```python
from build123d import *

# Parameters (mm, degrees)
SM_BASE_FLANGE_1_DEPTH = 113
EXTRUDE_1_DEPTH        = 4
HOLE_WIZARD_M3_1_D     = 2.5
SKETCH_10_R            = 11
CUT_EXTRUDE_1_DEPTH    = 2
HOLE_WIZARD_M3_2_D     = 2.5


# Sheet-metal steps are written as plain solids
with BuildPart() as part:
    # Sketch 1 → 基体-法兰1 (new body)
    with BuildSketch(Plane.XY):
        with BuildLine():
            Line((104, 47.58), (3.5, 47.58))
            ThreePointArc((3.5, 47.58), (1.025126266, 46.554873734), (0, 44.08))
            Line((0, 44.08), (0, -44.08))
            ThreePointArc((0, -44.08), (1.025126266, -46.554873734), (3.5, -47.58))
            Line((3.5, -47.58), (104, -47.58))
            Line((104, -47.58), (104, -45.58))
            Line((104, -45.58), (3.5, -45.58))
            ThreePointArc((3.5, -45.58), (2.439339828, -45.140660172), (2, -44.08))
            Line((2, -44.08), (2, 44.08))
            ThreePointArc((2, 44.08), (2.439339828, 45.140660172), (3.5, 45.58))
            Line((3.5, 45.58), (104, 45.58))
            Line((104, 45.58), (104, 47.58))
        make_face()
    extrude(amount=SM_BASE_FLANGE_1_DEPTH)

    # 草图6 → 凸台-拉伸1 (add)
    with BuildSketch(Plane.XY):
        with BuildLine():
            Line((104, 45.58), (3.5, 45.58))
            ThreePointArc((3.5, 45.58), (2.439339828, 45.140660172), (2, 44.08))
            Line((2, 44.08), (2, -44.08))
            ThreePointArc((2, -44.08), (2.439339828, -45.140660172), (3.5, -45.58))
            Line((3.5, -45.58), (104, -45.58))
            Line((104, -45.58), (104, 45.58))
        make_face()
    extrude(amount=EXTRUDE_1_DEPTH)

    # M3 螺纹孔1 (through all)
    with Locations(Plane(origin=(0, -47.58, 0), x_dir=(-1, 0, 0), z_dir=(0, -1, 0))):
        with Locations((-83.7, -100.6), (-96.2, -100.6)):
            Hole(HOLE_WIZARD_M3_1_D / 2)

    # 草图10 → 切除-拉伸1 (cut)
    with BuildSketch(Plane.ZY):
        with Locations(Location((47.4, -14.64, 0), (0, 0, 270))):
            Circle(SKETCH_10_R)
    extrude(amount=-CUT_EXTRUDE_1_DEPTH, mode=Mode.SUBTRACT)

    # M3 螺纹孔2 (through all)
    with Locations(Plane.XY.offset(4)):
        with Locations((41.5, 12.5), (66.5, 12.5), (66.5, -12.5), (41.5, -12.5)):
            Hole(HOLE_WIZARD_M3_2_D / 2)


solid = part.part
```
Geometry check sheet. Reference: the model listing, model coordinates, mm. A direction names the side the tool comes from. Give positions to 0.01 mm unless a question says otherwise; leave off trailing zeros. Order: outer loops, then holes, each group sorted by start corner. A loop starts at its lowest first (then second) coordinate and runs counter-clockwise, first axis right, second up. Notation, with made-up numbers: (-2, 80) - (39, 80) arc R12 cw to (39, 87) - close; hole circle Ø9 at (76.5, -6). An arc over 180 degrees is marked (long way). Write item = value, one per line. Start each with the question number.
1) Section check A-A (x = 14). Enter the section's corners in (y, z).
2) Gauge pin test, flat ends, axial feed: pin 1 Ø4 at (x, y) = (42, 26) entering from -Z; pin 2 Ø1.5 at (x, z) = (83.7, 100.6) entering from +Y; pin 3 Ø6 at (y, z) = (16.5, 52.5) entering from +X; pin 4 Ø3 at (x, y) = (66.5, 12.5) entering from +Z. Record the tip position at first contact, or that the pin passes through.
3) Section check D-D (y = -28). Enter the section's corners in (x, z), then the cut area to 3 significant figures.
4) Scan lines: L1, parallel to Y at x = 41.5, z = 2.65; L2, parallel to Y at x = 35.5, z = 36; L3, parallel to Z at x = 0.8, y = -14.64. Record each from-to range of solid material in increasing order.
5) Draft check along Y on faces 1 (the flat face through (2, -1, 58)), 2 (the cylindrical face through (1.05, 46.58, 55.71)), 3 (the cylindrical face through (0.99, -12.26, 36.66)), 4 (the flat face through (51, 1, 0)). Enter one of: released by +Y, released by -Y, zero draft, split by the parting line, or undercut.
6) Section check B-B (y = -5.5). Enter the section's corners in (x, z), then the cut area to 3 significant figures.
7) Section check C-C (z = 26.5). Enter the section's corners in (x, y).
8) Access from +Z, -Z, +X, -X, +Y, -Y to the whole of each face (thin tool, end or side, straight path). Record for faces 5 (the flat face through (54, -45.58, 58)), 6 (the flat face through (53, -47.58, 56)).
Geometry check:
q1.outline = (-47.58, 0) - (47.58, 0) - (47.58, 113) - (45.58, 113) - (45.58, 4) - (-45.58, 4) - (-45.58, 113) - (-47.58, 113) - close
q2.pin_1 = 0
q2.pin_2 = through
q2.pin_3 = 2
q2.pin_4 = 4
q3.outline = (0, 0) - (104, 0) - (104, 4) - (2, 4) - (2, 113) - (0, 113) - close
q3.area = 634 mm2
q4.L1 = -47.58 to -13.75, -11.25 to 11.25, 13.75 to 47.58
q4.L2 = -47.58 to -45.58, 45.58 to 47.58
q4.L3 = 0 to 36.4, 58.4 to 113
q5.face_1 = undercut
q5.face_2 = released by +Y
q5.face_3 = undercut
q5.face_4 = zero draft
q6.outline = (0, 0) - (104, 0) - (104, 4) - (2, 4) - (2, 41.28) - (0, 41.28) - close; (0, 53.52) - (2, 53.52) - (2, 113) - (0, 113) - close
q6.area = 610 mm2
q7.outline = (0, -44.08) arc R3.5 ccw to (3.5, -47.58) - (104, -47.58) - (104, -45.58) - (3.5, -45.58) arc R1.5 cw to (2, -44.08) - (2, 44.08) arc R1.5 cw to (3.5, 45.58) - (104, 45.58) - (104, 47.58) - (3.5, 47.58) arc R3.5 ccw to (0, 44.08) - close
q8.face_5 = +Z, +X
q8.face_6 = +Z, -Z, +X, -X, -Y
